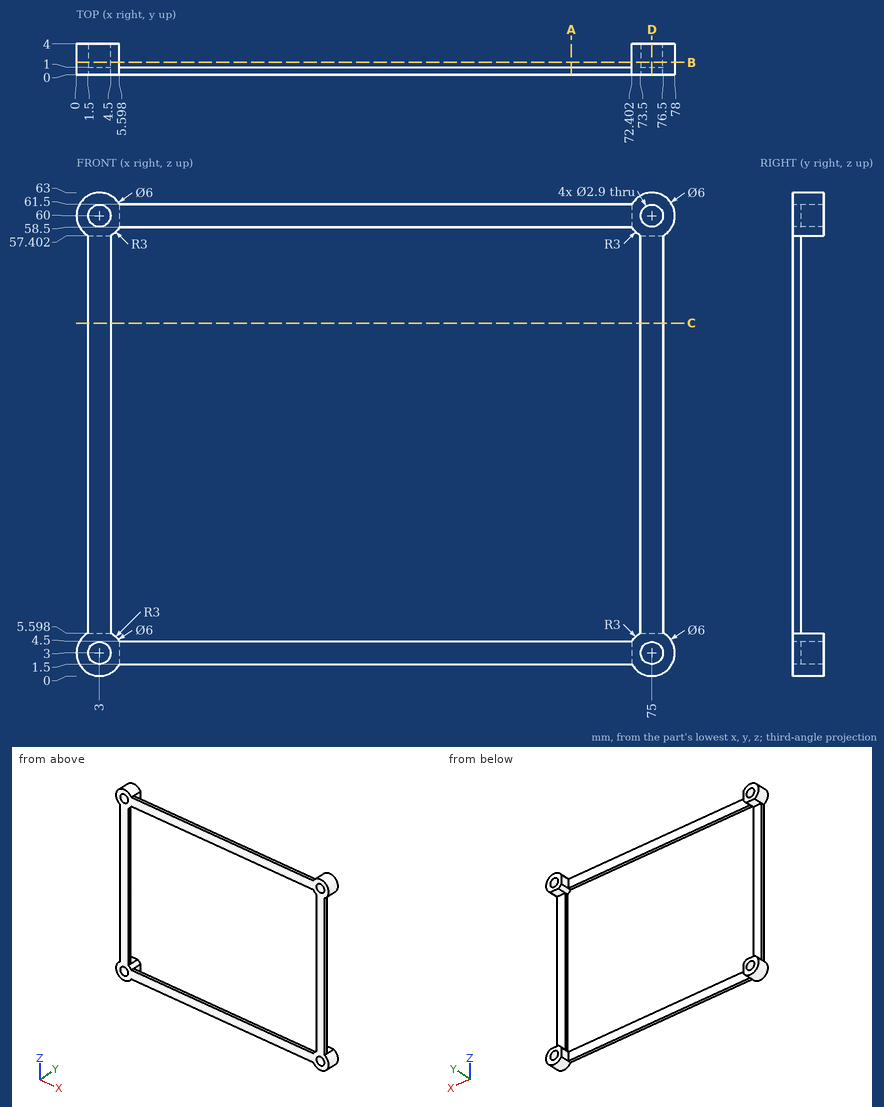
Geometry: see drawing. Coordinates: mm, zero at the bounding-box minimum. Coordinates: 2 decimals unless noted, no trailing zeros. Loops run counter-clockwise (first coordinate to the right, second up) from the corner with the lowest first, then second, coordinate; pieces in that order, holes last. Notation, with made-up numbers: (80.25, -3.5) - (102.25, -3.5) arc R26 ccw to (102.25, 24.5) - close; hole circle Ø1 at (75.25, 42.25). An arc over 180 degrees is marked (long way). Put each result on its own line as item: value. Start each with the question number.
Q1. Pin query (flat end, axial travel): pin 1 Ø0.8 at (x, y) = (31.5, 0.5) entering from -Z; pin 2 Ø1.5 at (y, z) = (1, 9) entering from -X; pin 3 Ø0.8 at (y, z) = (0.5, 37) entering from +X. Return the tip coordinate at first contact, or that it passes through.
Q2. Cut plane A-A, the plane x = 64.5. Return loops of the section in (y, z), and give its area (3 significant figures).
Q3. Cut plane B-B, the plane y = 1.6. Return loops of the section in (x, z).
Q4. Line query: line 1 (Z direction, x = 75, y = 3); line 2 (Z direction, x = 50.5, y = 0.85); line 3 (X direction, y = 0.6, z = 9.5). Output: solid intervals per line, ascending.
Q5. Cut plane D-D, the plane x = 75. Return loops of the section in (y, z), and give its area (3 significant figures).
Q6. Cut plane C-C, the plane z = 46. Return loops of the section in (x, y), and give its area (3 significant figures).
Filled sheet:
1. pin 1: z = 1.5
1. pin 2: x = 1.5
1. pin 3: x = 76.5
2. outline: (0, 1.5) - (1, 1.5) - (1, 4.5) - (0, 4.5) - close; (0, 58.5) - (1, 58.5) - (1, 61.5) - (0, 61.5) - close
2. area: 6.00 mm²
3. outline: (1.5, 5.6) arc R3 ccw (long way) to (5.6, 1.5) - (5.6, 4.5) arc R3 ccw to (4.5, 5.6) - close; (1.5, 57.4) - (4.5, 57.4) arc R3 ccw to (5.6, 58.5) - (5.6, 61.5) arc R3 ccw (long way) to start; (72.4, 1.5) arc R3 ccw (long way) to (76.5, 5.6) - (73.5, 5.6) arc R3 ccw to (72.4, 4.5) - close; (72.4, 58.5) arc R3 ccw to (73.5, 57.4) - (76.5, 57.4) arc R3 ccw (long way) to (72.4, 61.5) - close; hole circle Ø2.9 at (3, 3); hole circle Ø2.9 at (3, 60); hole circle Ø2.9 at (75, 3); hole circle Ø2.9 at (75, 60)
4. line 1: 0 to 1.55, 4.45 to 5.6, 57.4 to 58.55, 61.45 to 63
4. line 2: 1.5 to 4.5, 58.5 to 61.5
4. line 3: 1.5 to 4.5, 73.5 to 76.5
5. outline: (0, 0) - (4, 0) - (4, 1.55) - (0, 1.55) - close; (0, 4.45) - (4, 4.45) - (4, 5.6) - (1, 5.6) - (1, 57.4) - (4, 57.4) - (4, 58.55) - (0, 58.55) - close; (0, 61.45) - (4, 61.45) - (4, 63) - (0, 63) - close
5. area: 73.4 mm²
6. outline: (1.5, 0) - (4.5, 0) - (4.5, 1) - (1.5, 1) - close; (73.5, 0) - (76.5, 0) - (76.5, 1) - (73.5, 1) - close
6. area: 6.00 mm²
